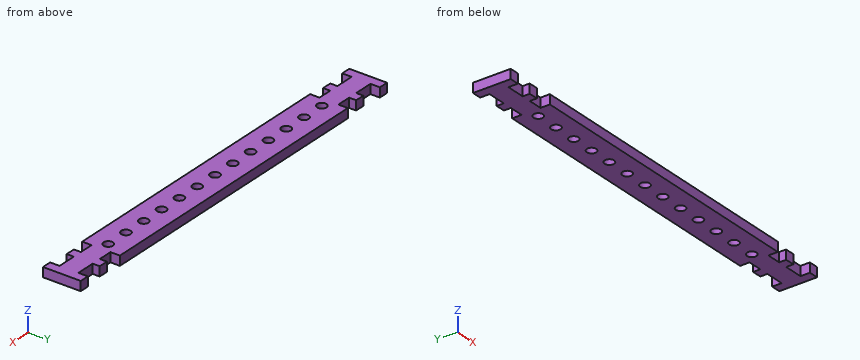
```python
from build123d import *

# Parameters (mm, degrees)
SKETCH_1_R      = 1.000000004
EXTRUDE_1_DEPTH = 2


with BuildPart() as part:
    # 草图1 → 凸台-拉伸1 (new body)
    with BuildSketch(Plane.XY):
        Polygon((-31.999107626, 4), (32.000892374, 4), (32.000892374, 2), (35.000892374, 2), (35.000892374, 3.5), (37.000892374, 3.5), (37.000892374, 2), (41.000892374, 2), (41.000892374, 4), (43.000892374, 4), (43.000892374, -4), (41.000892374, -4), (41.000892374, -2), (37.000892374, -2), (37.000892374, -3.5), (35.000892374, -3.5), (35.000892374, -2), (32.000892374, -2), (32.000892374, -4), (-31.999107626, -4), (-31.999107626, -2), (-34.999107626, -2), (-34.999107626, -3.5), (-36.999107626, -3.5), (-36.999107626, -2), (-40.999107626, -2), (-40.999107626, -4), (-42.999107626, -4), (-42.999107626, 4), (-40.999107626, 4), (-40.999107626, 2), (-36.999107626, 2), (-36.999107626, 3.5), (-34.999107626, 3.5), (-34.999107626, 2), (-31.999107626, 2), align=None)
        with Locations((0.000892374, 0)):
            Circle(SKETCH_1_R, mode=Mode.SUBTRACT)
        with Locations((5.000892374, 0)):
            Circle(SKETCH_1_R, mode=Mode.SUBTRACT)
        with Locations((10.000892374, 0)):
            Circle(SKETCH_1_R, mode=Mode.SUBTRACT)
        with Locations((15.000892374, 0)):
            Circle(SKETCH_1_R, mode=Mode.SUBTRACT)
        with Locations((20.000892374, 0)):
            Circle(SKETCH_1_R, mode=Mode.SUBTRACT)
        with Locations((25.000892374, 0)):
            Circle(SKETCH_1_R, mode=Mode.SUBTRACT)
        with Locations((30.000892374, 0)):
            Circle(SKETCH_1_R, mode=Mode.SUBTRACT)
        with Locations((-4.999107626, 0)):
            Circle(SKETCH_1_R, mode=Mode.SUBTRACT)
        with Locations((-9.999107626, 0)):
            Circle(SKETCH_1_R, mode=Mode.SUBTRACT)
        with Locations((-14.999107626, 0)):
            Circle(SKETCH_1_R, mode=Mode.SUBTRACT)
        with Locations((-19.999107626, 0)):
            Circle(SKETCH_1_R, mode=Mode.SUBTRACT)
        with Locations((-24.999107626, 0)):
            Circle(SKETCH_1_R, mode=Mode.SUBTRACT)
        with Locations((-29.999107626, 0)):
            Circle(SKETCH_1_R, mode=Mode.SUBTRACT)
    extrude(amount=EXTRUDE_1_DEPTH)


solid = part.part
```
Can you work these out from the model? Positions are in its coordinate system, mm. Give positions to 0.01 mm unless a question says otherwise; leave off trailing zeros. Write item = value, one per line. Start each with the question number.
1. Please list where these lines run through material, in increasing order: line 1 (X direction, y = -3, z = 0.4); line 2 (Y direction, x = 34.5, z = 1).
2. Imagine slicing it at A-A (y = 0). Count the separate pieces of the cut face and the enclosed holes in it, and give its area (3 significant figures).
3. For pin 1 (1 mm diameter, centred on x = 34, z = 1, fed in from -Y); pin 2 (1 mm diameter, centred on x = -36, z = 1.5, fed in from -Y); pin 3 (1 mm diameter, centred on x = 15.5, y = -1.5, fed in from -Z); pin 4 (1 mm diameter, centred on x = 33, z = 0.5, fed in from +Y), each with a flat end and sliding along its axis, tell me the tip position at first contact or that it passes through.
Worked answers:
q1.line_1 = -43 to -41, -37 to -35, -32 to 32, 35 to 37, 41 to 43
q1.line_2 = -2 to 2
q2.separate_pieces = 14
q2.enclosed_holes = 0
q2.area = 120 mm2
q3.pin_1 = -2
q3.pin_2 = -3.5
q3.pin_3 = 0
q3.pin_4 = 2
